Input: part model. Units: mm. Frame: model coordinates. Face numbers are marked on the shaded views. A direction names the side the tool comes from. Give positions to 0.01 mm unless a question says otherwise; leave off trailing zeros. Order: outer loops, then holes, each group sorted by start corner. A loop starts at its lowest first (then second) coordinate and runs counter-clockwise, first axis right, second up. Notation, with made-up numbers: (-39.75, 75.5) - (-35.75, 75.5) arc R24 ccw to (-35.75, 94.5) - close; hole circle Ø7 at (24, 67). An arc over 180 degrees is marked (long way). Answer in a Markdown table with one row per item. Add a question column.
1. Section query A-A on x = 0. Return loops of the section in (y, z), and give its area (3 significant figures).
2. Section query C-C on y = 11.5. Return loops of the section in (x, z), and give its area (3 significant figures).
3. Section query D-D on x = -49.5. Return loops of the section in (y, z).
4. Ray query, line 1 (Y direction, x = -29, z = -26); line 2 (Z direction, x = 12, y = 27); line 3 (Z direction, x = 1, y = 22). Return the intervals inside material, ascending. Write a range as [from, to].
5. Access query for the marked faces 1 and 2. Directions: +Z, -Z, +X, -X, +Y, -Y. A direction counts if a zero-diameter tool reaches every point of the face in a straight line with its end or side. Return the directions, or none.
6. Mould query, pull axis X, two halves, no side actions, for the marked faces 3, 4, 5 and 6. Classes: released by +X, released by -X, zero draft, split by the parting line, or undercut.
7. Section query B-B on z = 0. Return loops of the section in (x, y).
8. Contact query for flat-ended pins moving along their axis: pin 1 (2.5 mm diameter, centred on x = 30.26, z = 12.14, fed in from -Y); pin 2 (1.5 mm diameter, centred on x = -48, z = 26.5, fed in from -Y); pin 3 (12 mm diameter, centred on y = 22, z = 11.5, fed in from +X); pin 4 (1.2 mm diameter, centred on x = -16.5, z = -13, fed in from -Y). Output: stop coordinate, or through.
```python
from build123d import *

# Parameters (mm, degrees)
CROQUIS1_R              = 27.5
SALIENTE_EXTRUIR1_DEPTH = 20
CROQUIS3_R              = 5.5
CORTAR_EXTRUIR1_DEPTH   = 10
CROQUIS4_R              = 2
CORTAR_EXTRUIR2_DEPTH   = 10
CROQUIS5_R              = 60
SALIENTE_EXTRUIR2_DEPTH = 13
CORTAR_EXTRUIR3_DEPTH   = 92.043945433
CROQUIS7_R              = 2.186456698
CORTAR_EXTRUIR4_DEPTH   = 88.177978871


with BuildPart() as part:
    # Croquis1 → Saliente-Extruir1 (new body)
    with BuildSketch(Plane(origin=(0, 0, 0), x_dir=(1, 0, 0), z_dir=(0, 1, 0))):
        with Locations(Location((0, 0, 0), (0, 0, 270))):
            Circle(CROQUIS1_R)
    extrude(amount=SALIENTE_EXTRUIR1_DEPTH)

    # Croquis3 → Cortar-Extruir1 (cut)
    with BuildSketch(Plane(origin=(0, 20, 0), x_dir=(1, 0, 0), z_dir=(0, 1, 0))):
        with Locations(Location((0, 0, 0), (0, 0, 270))):
            Circle(CROQUIS3_R)
    extrude(amount=-CORTAR_EXTRUIR1_DEPTH, mode=Mode.SUBTRACT)

    # Croquis4 → Cortar-Extruir2 (cut)
    with BuildSketch(Plane.XZ):
        with Locations(Location((12.224300889, -15.829291449, 0), (0, 0, 270))):
            Circle(CROQUIS4_R)
        with Locations(Location((-15.829291449, -12.224300889, 0), (0, 0, 270))):
            Circle(CROQUIS4_R)
        with Locations(Location((-12.224300889, 15.829291449, 0), (0, 0, 270))):
            Circle(CROQUIS4_R)
        with Locations(Location((15.829291449, 12.224300889, 0), (0, 0, 270))):
            Circle(CROQUIS4_R)
    extrude(amount=-CORTAR_EXTRUIR2_DEPTH, mode=Mode.SUBTRACT)

    # Croquis5 → Saliente-Extruir2 (add)
    with BuildSketch(Plane(origin=(0, 20, 0), x_dir=(1, 0, 0), z_dir=(0, 1, 0))):
        with Locations(Location((0, 0, 0), (0, 0, 90))):
            Circle(CROQUIS5_R)
    extrude(amount=SALIENTE_EXTRUIR2_DEPTH)

    # Croquis6 → Cortar-Extruir3 (cut, through all)
    with BuildSketch(Plane(origin=(0, 33, 0), x_dir=(1, 0, 0), z_dir=(0, 1, 0))):
        Polygon((28.483293317, 26.915833338), (21.280272026, 22.80257149), (30.330623274, 6.953866704), (37.533644565, 11.067128551), align=None)
    extrude(amount=-CORTAR_EXTRUIR3_DEPTH, mode=Mode.SUBTRACT)

    # Croquis7 → Cortar-Extruir4 (cut, through all)
    with BuildSketch(Plane.XZ.offset(-20)):
        with Locations(Location((-30.256887418, -12.141762544, 0), (0, 0, 270))):
            Circle(CROQUIS7_R)
        with Locations(Location((-12.141762544, 30.256887418, 0), (0, 0, 270))):
            Circle(CROQUIS7_R)
        with Locations(Location((30.256887418, 12.141762544, 0), (0, 0, 270))):
            Circle(CROQUIS7_R)
        with Locations(Location((12.141762544, -30.256887418, 0), (0, 0, 270))):
            Circle(CROQUIS7_R)
    extrude(amount=-CORTAR_EXTRUIR4_DEPTH, mode=Mode.SUBTRACT)


solid = part.part
```
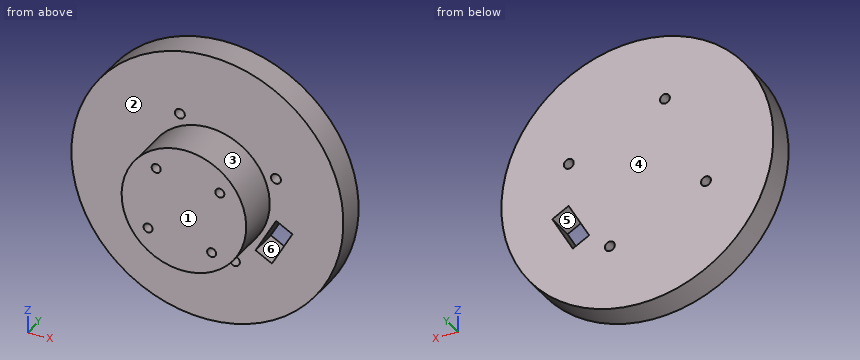
Answer:
| question | item | result |
|---|---|---|
| 1 | outline | (0, -27.5) - (20, -27.5) - (20, -60) - (33, -60) - (33, 60) - (20, 60) - (20, 27.5) - (0, 27.5) - close; hole (10, -5.5) - (20, -5.5) - (20, 5.5) - (10, 5.5) - close |
| 1 | area | 2,550 mm² |
| 2 | outline | circle Ø55 at (0, 0); hole circle Ø11 at (0, 0) |
| 2 | area | 2,280 mm² |
| 3 | outline | (20, -33.91) - (33, -33.91) - (33, 33.91) - (20, 33.91) - close |
| 4 | line 1 | y = [20, 33] |
| 4 | line 2 | z = [-58.79, -32.44], [-28.08, 58.79] |
| 4 | line 3 | z = [-59.99, 59.99] |
| 5 | face 1 | +Z, -Z, +X, -X, -Y |
| 5 | face 2 | -Y |
| 6 | face 3 | split by the parting line |
| 6 | face 4 | zero draft |
| 6 | face 5 | undercut |
| 6 | face 6 | undercut |
| 7 | outline | (-60, 20) - (-27.5, 20) - (-27.5, 0) - (27.5, 0) - (27.5, 20) - (60, 20) - (60, 33) - (-60, 33) - close; hole (-5.5, 10) - (5.5, 10) - (5.5, 20) - (-5.5, 20) - close |
| 8 | pin 1 | passes through |
| 8 | pin 2 | stops at y = 20 |
| 8 | pin 3 | stops at x = 59.75 |
| 8 | pin 4 | stops at y = 10 |
